CAD build for the part. Positions are in the model's coordinates, mm. A direction names the side the tool comes from. Coordinates: 2 decimals unless noted, no trailing zeros. Order: outer loops, then holes, each group sorted by start corner. A loop starts at its lowest first (then second) coordinate and runs counter-clockwise, first axis right, second up. Notation, with made-up numbers: M 40,89.5 L 45,89.5 A19 cw 45,117.5 Z; hole C 12.25,-17 d1. An arc over 180 degrees is marked long. Write item = value, one per line.
Autodesk Inventor part; units mm, degrees
ref_plane "Work Plane1" through (0, 0, 6) normal (0, 0, 1) x (1, 0, 0)
ref_plane "Work Plane4" through (-8, 19, 6) normal (0, 1, 0) x (1, 0, 0)
ref_plane "Work Plane3" through (8, 0, 6) normal (1, 0, 0) x (0, 0, -1)
sketch "Sketch1" plane through (0, 0, 0) normal (0, 0, 1) x (1, 0, 0)
  circle A0 centre (0, 0) radius 3.25
  circle A1 centre (0, 0) radius 8
  dimension "d0" = 6.5
  dimension "d1" = 16
extrude "Extrusion1" add sketch "Sketch1" along normal blind 6
sketch "Sketch2" plane through (0, 0, 0) normal (1, 0, 0) x (0, 1, 0)
  circle A0 centre (0, 2.5) radius 1.25
  point P0 (0, 0)
  dimension "d4" = 2.5
extrude "Extrusion2" cut sketch "Sketch2" against normal blind 20
ref_plane "Work Plane1" through (0, 0, 6) normal (0, 0, 1) x (1, 0, 0)
sketch "Sketch3" plane through (0, 0, 6) normal (0, 0, 1) x (1, 0, 0)
  circle A0 centre (0, 0) radius 7.5
  line L0 (-8, 0) -> (8, 0)
  line L1 (8, 0) -> (8, 19)
  line L2 (8, 19) -> (-8, 19)
  line L3 (-8, 19) -> (-8, 0)
  dimension "d9" = 16
  dimension "d10" = 19
  dimension "d11" = 8
  dimension "d17" = 0
extrude "Extrusion3" add sketch "Sketch3" against normal blind 6 contours L0 A0 | A0 L0 L3 L2 L1 picked at (-1.3085, 5.1375)
sketch "Sketch4" plane through (0, 0, 0) normal (0, 0, -1) x (-1, 0, 0)
  line L0 (8, 0) -> (8, 19)
  line L1 (-8, 19) -> (8, 19)
  line L2 (8, 19) -> (8, 11)
  line L3 (8, 11) -> (-8, 11)
  line L4 (-8, 11) -> (-8, 19)
  dimension "d14" = 8
extrude "Extrusion4" add sketch "Sketch4" along normal blind 10
ref_plane "Work Plane4" through (-8, 19, 6) normal (0, 1, 0) x (1, 0, 0)
sketch "Sketch5" plane through (-8, 19, 6) normal (0, 1, 0) x (1, 0, 0)
  line L0 (16, 0) -> (16, 16)
  line L1 (0, 16) -> (16, 16)
  circle A0 centre (8.9, 11) radius 2.2
  point P0 (8, 6)
  dimension "d18" = 4.4
  dimension "d19" = 7.1
  dimension "d20" = 5
extrude "Extrusion5" cut sketch "Sketch5" against normal blind 10
ref_plane "Work Plane3" through (8, 0, 6) normal (1, 0, 0) x (0, 0, -1)
sketch "Sketch6" plane through (8, 0, 6) normal (1, 0, 0) x (0, 0, -1)
  line L0 (16, 19) -> (16, 11)
  line L1 (0, 19) -> (16, 19)
  line L2 (0, 19) -> (16, 19)
  line L3 (16, 19) -> (16, 11)
  line L4 (16, 11) -> (0, 11)
  line L5 (0, 11) -> (0, 19)
extrude "Extrusion6" add sketch "Sketch6" along normal blind 2
ref_plane "Work Plane5" through (-8, 19, 6) normal (0, 1, 0) x (1, 0, 0)
sketch "Sketch7" plane through (-8, 19, 6) normal (0, 1, 0) x (1, 0, 0)
  circle A0 centre (8.9, 11) radius 2.2
  line L0 (18, 0) -> (0, 0)
  line L1 (18, 16) -> (18, 0)
  line L2 (0, 16) -> (18, 16)
  line L3 (17, 0) -> (1, 0)
  line L4 (1, 0) -> (1, 16)
  line L5 (1, 16) -> (17, 16)
  line L6 (17, 16) -> (17, 0)
  point P0 (8, 6)
  dimension "d25" = 16
  dimension "d26" = 1
extrude "Extrusion7" cut sketch "Sketch7" against normal blind 3 contours L0 L4 L2 L6
sketch "Sketch8" plane through (0, 0, 0) normal (0, 0, -1) x (-1, 0, 0)
  arc A0 (-3.75, 0) -> (3.75, 0) centre (0, 0) ccw
  circle A1 centre (0, 0) radius 3.25
  dimension "d29" = 6.5
extrude "Extrusion8" cut sketch "Sketch8" against normal through all
ref_plane "Work Plane2" through (-8, 0, 0.75) normal (-1, 0, 0) x (0, 0, 1)
sketch "Sketch9" plane through (-8, 0, 0.75) normal (-1, 0, 0) x (0, 0, 1)
  line L0 (3.5, 0) -> (0, 0)
  circle A0 centre (1.75, 0) radius 1.25
  point P0 (-0.75, 0)
  dimension "d35" = 2.5
extrude "Extrusion9" cut sketch "Sketch9" against normal blind 8
sketch "Sketch11" plane through (0, 0, -10) normal (0, 0, -1) x (-1, 0, 0)
  line L0 (-9, 16) -> (-9, 19)
  line L1 (8, 19) -> (-10, 19)
  line L2 (-10, 11) -> (-10, 19)
  line L3 (8, 11) -> (-10, 11)
  line L4 (8, 11) -> (8, 19)
  line L5 (8, 19) -> (7, 19)
  line L6 (7, 19) -> (7, 16)
  line L7 (7, 16) -> (-9, 16)
  point P0 (0, 0)
  point P1 (-8, 19)
  point P2 (-8, 11)
extrude "Extrusion10" add sketch "Sketch11" along normal blind 6 contours L7 L6 L1 L4 L3 L2 L0
sketch "Sketch13" plane through (0, 0, 0) normal (0, 0, -1) x (-1, 0, 0)
  circle A0 centre (0, 0) radius 3.25
  line L0 (8, 11) -> (-8, 11)
  line L1 (-8, 11) -> (-8, 0)
  arc A1 (-8, 0) -> (8, 0) centre (0, 0) ccw
  line L2 (8, 0) -> (8, 11)
extrude "Extrusion11" add sketch "Sketch13" along normal blind 16
sketch "Sketch15" plane through (8, 0, 6) normal (1, 0, 0) x (0, 0, -1)
  line L0 (0, 11) -> (16, 11)
  line L1 (16, 11) -> (16, -8.6618)
  line L2 (16, -8.6618) -> (0, -8.6618)
  line L3 (0, -8.6618) -> (0, 11)
  point P0 (6, 0)
  dimension "d43" = 16
extrude "Extrusion12" cut sketch "Sketch15" against normal blind 16
sketch "Sketch16" plane through (-8, 11, 6) normal (-1, 0, 0) x (0, 0, 1)
  line L0 (-22, -11) -> (-16, -11)
  circle A0 centre (-19, -11) radius 1.25
  point P0 (-6, -11)
  dimension "d46" = 2.5
extrude "Extrusion13" cut sketch "Sketch16" against normal blind 7
sketch "Sketch17" plane through (0, 0, 6) normal (0, 0, 1) x (1, 0, 0)
  line L0 (-8, 11) -> (10, 11)
  line L1 (10, 19) -> (10, 11)
  line L2 (10, 19) -> (9, 19)
  line L3 (9, 19) -> (9, 16)
  line L4 (9, 16) -> (-7, 16)
  line L5 (-7, 16) -> (-7, 19)
  line L6 (-7, 19) -> (-8, 19)
  line L7 (-8, 19) -> (-8, 11)
  point P0 (0, 0)
extrude "Extrusion14" cut sketch "Sketch17" against normal blind 6
fillet "Fillet9" radius 0.5 18 edges at (1, 11, 0) (-8, 15, 0) (10, 15, 0) (10, 11, -8) (0, 11, -10) (0, -8, -10) (-8, 5.5, -10) (8, 5.5, -10) (8, 11, -13) (9, 11, -16) (0, -8, -16) (-8, 9.5, -16) (8, 5.5, -16) (10, 15, -16) (-8, 11, -5) (-1.3, 11, -5) (3.25, 0, -10) (3.25, 0, -16)
properties part number "6mmRingBracketLeft"
(1) Pull direction Y, two halves, no side cores. Call faces 4 (the face through (3.247, -0.143, -12.965)), 5 (the face through (9.5, 19, -7.9)), 6 (the face through (1, 14, 0)): +Y half, -Y half, draft (parallel to the pull), parting line (faces both ways), or undercut.
Evaluation:
face_4 = undercut
face_5 = +Y half
face_6 = draft
(2) Wall check: line 1 (Y direction, x = 0, z = -13.8); line 2 (Z direction, x = 0.9, y = 13.35); line 3 (X direction, y = 16.25, z = -1.5). Give the ranges that are in metal, low to high. Write a range as from..to.
Evaluation:
line_1 = -8..-3.25, 3.25..16
line_2 = -16..-7.2, -2.8..0
line_3 = -8..-7, 9..10
(3) Slice it at D-D, the plane x = 0.9. State how many separate pieces and enclosed holes the cut face has, then the cut area to 3 significant figures.
Evaluation:
separate_pieces = 3
enclosed_holes = 0
area = 134 mm²
(4) Slice it at A-A, the plane z = -5. Write the cut outline in (x, y), then the cut area to 3 significant figures.
Evaluation:
outline = M -8,11.5 A0.5 ccw -7.5,11 L -1.8,11 A0.5 ccw -1.3,11.5 L -1.3,16 L -7,16 L -7,19 L -8,19 Z; M 3.1,11.5 A0.5 ccw 3.6,11 L 9.5,11 A0.5 ccw 10,11.5 L 10,19 L 9,19 L 9,16 L 3.1,16 Z
area = 73.8 mm²
(5) Slice it at B-B, the plane y = 13.5. Write the cut outline in (x, z).
Evaluation:
outline = M -8,-15.5 A0.5 ccw -7.5,-16 L 9.5,-16 A0.5 ccw 10,-15.5 L 10,-0.5 A0.5 ccw 9.5,0 L -7.5,0 A0.5 ccw -8,-0.5 Z; hole C 0.9,-5 d4.4
(6) Slice it at C-C, the plane z = -1. Write the cut outline in (x, y).
Evaluation:
outline = M -8,11.5 A0.5 ccw -7.5,11 L 9.5,11 A0.5 ccw 10,11.5 L 10,19 L 9,19 L 9,16 L -7,16 L -7,19 L -8,19 Z
(7) Pin check, flat tips, straight feed: pin 1 Ø8 at (y, z) = (-1.5, -6.5) entering from -X; pin 2 Ø3 at (x, y) = (-3.5, 6) entering from +Z; pin 3 Ø7 at (x, z) = (0.9, -5) entering from -Y. Stop position of each tip, or through.
Evaluation:
pin_1 = -7.97
pin_2 = -10
pin_3 = 11
(8) Tool access for faces 1 (the face through (2, 4, -10)), 2 (the face through (1, 16, -8)), 3 (the face through (8, 5, -13)): list every direction of +Z, -Z, +X, -X, +Y, -Y with a clear straight run to the whole face (end or side of a thin tool).
Evaluation:
face_1 = +Z, +X, -X, -Y
face_2 = +Z, -Z, +Y
face_3 = +Z, -Z, +X, -Y
